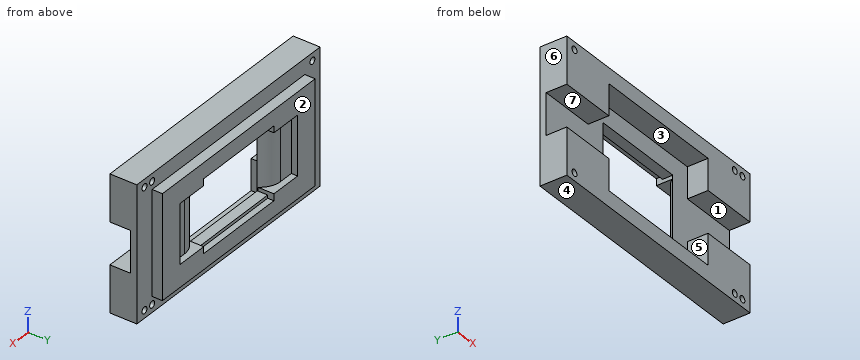
from build123d import *

# Parameters (mm, degrees)
BOSS_EXTRUDE3_DEPTH = 2
SKETCH1_6_W         = 100
SKETCH1_6_H         = 50
BOSS_EXTRUDE4_DEPTH = 5
SKETCH2_W           = 120
SKETCH2_H           = 65
SKETCH2_R           = 1.6
BOSS_EXTRUDE5_DEPTH = 13
SKETCH2_2_W         = 120
SKETCH2_2_H         = 65
SKETCH2_2_R         = 1.6
BOSS_EXTRUDE6_DEPTH = 3
CUT_EXTRUDE1_REACH  = 71.866
SKETCH7_W           = 43
SKETCH7_H           = 32
FILLET1_R           = 10
SKETCH8_W           = 38.5
SKETCH8_H           = 20
CUT_EXTRUDE2_DEPTH  = 10
SKETCH9_W           = 65
SKETCH9_H           = 50
CUT_EXTRUDE3_DEPTH  = 10


with BuildPart() as part:
    # Sketch1 → Boss-Extrude3 (new body)
    with BuildSketch(Plane(origin=(0, 0, 0), x_dir=(1, 0, 0), z_dir=(0, 1, 0))):
        Polygon((23, -14.25), (23, -17.5), (-23, -17.5), (-23, -14.25), (-38.5, -14.25), (-38.5, 14.25), (-23, 14.25), (-23, 17.5), (23, 17.5), (23, 14.25), (38.5, 14.25), (38.5, -14.25), align=None)
    extrude(amount=BOSS_EXTRUDE3_DEPTH)

    # Sketch1<6> → Boss-Extrude4 (add)
    with BuildSketch(Plane(origin=(0, 0, 0), x_dir=(1, 0, 0), z_dir=(0, 1, 0))):
        Rectangle(SKETCH1_6_W, SKETCH1_6_H)
        Polygon((23, -14.25), (23, -17.5), (-23, -17.5), (-23, -14.25), (-38.5, -14.25), (-38.5, 14.25), (-23, 14.25), (-23, 17.5), (23, 17.5), (23, 14.25), (38.5, 14.25), (38.5, -14.25), align=None, mode=Mode.SUBTRACT)
    extrude(amount=BOSS_EXTRUDE4_DEPTH)

    # Sketch2 → Boss-Extrude5 (add)
    with BuildSketch(Plane.XZ):
        Rectangle(SKETCH2_W, SKETCH2_H)
        with Locations(Location((-55, 28.75, 0), (0, 0, 90))):
            Circle(SKETCH2_R, mode=Mode.SUBTRACT)
        with Locations(Location((55, 28.75, 0), (0, 0, 90))):
            Circle(SKETCH2_R, mode=Mode.SUBTRACT)
        with Locations(Location((55, -28.75, 0), (0, 0, 90))):
            Circle(SKETCH2_R, mode=Mode.SUBTRACT)
        with Locations(Location((-55, -28.75, 0), (0, 0, 90))):
            Circle(SKETCH2_R, mode=Mode.SUBTRACT)
        with Locations(Location((50, 28.75, 0), (0, 0, 90))):
            Circle(SKETCH2_R, mode=Mode.SUBTRACT)
        with Locations(Location((50, -28.75, 0), (0, 0, 90))):
            Circle(SKETCH2_R, mode=Mode.SUBTRACT)
    extrude(amount=BOSS_EXTRUDE5_DEPTH)

    # Sketch2<2> → Boss-Extrude6 (add)
    with BuildSketch(Plane.XZ):
        Rectangle(SKETCH2_2_W, SKETCH2_2_H)
        with Locations(Location((-55, 28.75, 0), (0, 0, 90))):
            Circle(SKETCH2_2_R, mode=Mode.SUBTRACT)
        with Locations(Location((55, 28.75, 0), (0, 0, 90))):
            Circle(SKETCH2_2_R, mode=Mode.SUBTRACT)
        with Locations(Location((55, -28.75, 0), (0, 0, 90))):
            Circle(SKETCH2_2_R, mode=Mode.SUBTRACT)
        with Locations(Location((-55, -28.75, 0), (0, 0, 90))):
            Circle(SKETCH2_2_R, mode=Mode.SUBTRACT)
        with Locations(Location((50, 28.75, 0), (0, 0, 90))):
            Circle(SKETCH2_2_R, mode=Mode.SUBTRACT)
        with Locations(Location((50, -28.75, 0), (0, 0, 90))):
            Circle(SKETCH2_2_R, mode=Mode.SUBTRACT)
    extrude(amount=BOSS_EXTRUDE6_DEPTH)

    # Sketch7 → Cut-Extrude1 (cut, up to next)
    with BuildSketch(Plane(origin=(0, 2, 0), x_dir=(1, 0, 0), z_dir=(0, 1, 0)), mode=Mode.PRIVATE) as cut_extrude1_sk1:
        Rectangle(SKETCH7_W, SKETCH7_H)
    cut_extrude1_tool1 = extrude(cut_extrude1_sk1.sketch, amount=-CUT_EXTRUDE1_REACH, mode=Mode.PRIVATE) & part.part
    add(cut_extrude1_tool1.solids().sort_by_distance((0, 2, 0))[0], mode=Mode.SUBTRACT)

    # Fillet1
    # the kernel refuses this fillet: 10 mm, written as the material it takes off along each edge
    with BuildSketch(Plane(origin=(-21.5, 2, 16), x_dir=(0, -1, 0), z_dir=(0, 0, -1))) as fillet1_piece_1_section:
        with BuildLine():
            CenterArc((FILLET1_R, FILLET1_R), FILLET1_R, 180, 90)
            Line((0, FILLET1_R), (0, 0))
            Line((0, 0), (FILLET1_R, 0))
        make_face()
    fillet1_piece_1 = extrude(amount=32, mode=Mode.PRIVATE)
    fillet1_piece_1 = split(fillet1_piece_1, bisect_by=Plane(origin=(-23, -2.387167078, 15.125), z_dir=(1, 0, 0)), keep=Keep.TOP, mode=Mode.PRIVATE)
    add(fillet1_piece_1, mode=Mode.SUBTRACT)
    with BuildSketch(Plane(origin=(-21.5, 2, 41), x_dir=(0, -1, 0), z_dir=(0, 0, -1))) as fillet1_piece_2_section:
        with BuildLine():
            CenterArc((FILLET1_R, FILLET1_R), FILLET1_R, 180, 90)
            Line((0, FILLET1_R), (0, 0))
            Line((0, 0), (FILLET1_R, 0))
        make_face()
    fillet1_piece_2 = extrude(amount=82, mode=Mode.PRIVATE)
    fillet1_piece_2 = split(fillet1_piece_2, bisect_by=Plane(origin=(-23.780995079, -0.852225246, -14.25), z_dir=(0, 0, 1)), keep=Keep.TOP, mode=Mode.PRIVATE)
    fillet1_piece_2 = split(fillet1_piece_2, bisect_by=Plane(origin=(-23.780995079, -0.852225246, 14.25), z_dir=(0, 0, -1)), keep=Keep.TOP, mode=Mode.PRIVATE)
    add(fillet1_piece_2, mode=Mode.SUBTRACT)
    with BuildSketch(Plane(origin=(21.5, 2, -16), x_dir=(0, -1, 0), z_dir=(0, 0, 1))) as fillet1_piece_3_section:
        with BuildLine():
            CenterArc((FILLET1_R, FILLET1_R), FILLET1_R, 180, 90)
            Line((0, FILLET1_R), (0, 0))
            Line((0, 0), (FILLET1_R, 0))
        make_face()
    fillet1_piece_3 = extrude(amount=32, mode=Mode.PRIVATE)
    fillet1_piece_3 = split(fillet1_piece_3, bisect_by=Plane(origin=(23, -2.387167078, -15.125), z_dir=(-1, 0, 0)), keep=Keep.TOP, mode=Mode.PRIVATE)
    add(fillet1_piece_3, mode=Mode.SUBTRACT)
    with BuildSketch(Plane(origin=(21.5, 2, -41), x_dir=(0, -1, 0), z_dir=(0, 0, 1))) as fillet1_piece_4_section:
        with BuildLine():
            CenterArc((FILLET1_R, FILLET1_R), FILLET1_R, 180, 90)
            Line((0, FILLET1_R), (0, 0))
            Line((0, 0), (FILLET1_R, 0))
        make_face()
    fillet1_piece_4 = extrude(amount=82, mode=Mode.PRIVATE)
    fillet1_piece_4 = split(fillet1_piece_4, bisect_by=Plane(origin=(23.780995079, -0.852225246, 14.25), z_dir=(0, 0, -1)), keep=Keep.TOP, mode=Mode.PRIVATE)
    fillet1_piece_4 = split(fillet1_piece_4, bisect_by=Plane(origin=(23.780995079, -0.852225246, -14.25), z_dir=(0, 0, 1)), keep=Keep.TOP, mode=Mode.PRIVATE)
    add(fillet1_piece_4, mode=Mode.SUBTRACT)

    # Sketch8 → Cut-Extrude2 (cut)
    with BuildSketch(Plane.XZ.offset(13)):
        with Locations((-40.75, 0)):
            Rectangle(SKETCH8_W, SKETCH8_H)
        with Locations((40.75, 0)):
            Rectangle(SKETCH8_W, SKETCH8_H)
    extrude(amount=-CUT_EXTRUDE2_DEPTH, mode=Mode.SUBTRACT)

    # Sketch9 → Cut-Extrude3 (cut)
    with BuildSketch(Plane(origin=(0, -13, 0), x_dir=(-1, 0, 0), z_dir=(0, -1, 0))):
        Rectangle(SKETCH9_W, SKETCH9_H)
    extrude(amount=-CUT_EXTRUDE3_DEPTH, mode=Mode.SUBTRACT)


solid = part.part
Geometry: final body of the model. Coordinates: model frame, mm. Face numbers are marked on the shaded views. A direction names the side the tool comes from. Coordinates: 2 decimals unless noted, no trailing zeros. Write each loop counter-clockwise with the first axis right and the second up, starting at its lowest first coordinate (ties: lowest second). Pieces come first, ordered by that corner, then holes. Notation, with made-up numbers: (67.5, 26) - (72.5, 26) arc R35 cw to (72.5, 60) - close; hole circle Ø2 at (-19.5, 57.5). An arc over 180 degrees is marked (long way). Return JSON: item names as keys, results as strings.
Item 1: Pull-direction query (Z, two-part tool) for the marked faces 4, 5, 6 and 7; classes: +Z half, -Z half, draft (parallel to the pull), parting line (faces both ways), or undercut.
Completed:
{"face 4": "-Z half", "face 5": "undercut", "face 6": "draft", "face 7": "undercut"}
Item 2: Section query C-C (z = 28.75). Output: boundary loops of the cut face in (x, y).
Completed:
{"outline": "(-60, -13) - (-56.6, -13) - (-56.6, 0) - (-60, 0) - close; (-53.4, -13) - (48.4, -13) - (48.4, 0) - (-53.4, 0) - close; (51.6, -13) - (53.4, -13) - (53.4, 0) - (51.6, 0) - close; (56.6, -13) - (60, -13) - (60, 0) - (56.6, 0) - close"}
Item 3: Pin query (flat end, axial travel): pin 1 Ø3 at (x, z) = (-55, -28.75) entering from -Y; pin 2 Ø2.5 at (y, z) = (4, 1) entering from -X; pin 3 Ø1.2 at (x, z) = (2.5, 16.5) entering from +Y; pin 4 Ø2.5 at (x, y) = (6, 2.5) entering from -Z. Return the tip coordinate at first contact, or that it passes through.
Completed:
{"pin 1": "passes through", "pin 2": "stops at x = -50", "pin 3": "stops at y = 2", "pin 4": "stops at z = -25"}
Item 4: Section query B-B (x = -1.5). Output: boundary loops of the cut face in (y, z).
Completed:
{"outline": "(-13, -32.5) - (0, -32.5) - (0, -25) - (5, -25) - (5, -17.5) - (2, -17.5) - (2, -16) - (-3, -16) - (-3, -25) - (-13, -25) - close; (-13, 25) - (-3, 25) - (-3, 16) - (2, 16) - (2, 17.5) - (5, 17.5) - (5, 25) - (0, 25) - (0, 32.5) - (-13, 32.5) - close"}
Item 5: Reachability of the marked faces 1, 2 and 3 from +Z, -Z, +X, -X, +Y, -Y: full face, straight path, thin tool, end or side. Return the list, or none.
Completed:
{"face 1": "+X, -X, -Y", "face 2": "+Z, -Z, +X, -X, +Y", "face 3": "-Y"}
Item 6: Section query A-A (y = -6.5). Output: boundary loops of the cut face in (x, z), and give its area (3 significant figures).
Completed:
{"outline": "(-60, -32.5) - (60, -32.5) - (60, -10) - (32.5, -10) - (32.5, -25) - (-32.5, -25) - (-32.5, -10) - (-60, -10) - close; (-60, 10) - (-32.5, 10) - (-32.5, 25) - (32.5, 25) - (32.5, 10) - (60, 10) - (60, 32.5) - (-60, 32.5) - close; hole circle Ø3.2 at (-55, -28.75); hole circle Ø3.2 at (-55, 28.75); hole circle Ø3.2 at (50, -28.75); hole circle Ø3.2 at (50, 28.75); hole circle Ø3.2 at (55, -28.75); hole circle Ø3.2 at (55, 28.75)", "area": "3,400 mm2"}
Item 7: Line query: L1, parallel to X at y = -2.5, z = -28.75; L2, parallel to Z at x = 55, y = -6.5; L3, parallel to Z at x = -4, y = -2.5. Output: solid intervals per line, ascending.
Completed:
{"L1": "x = -60 to -56.6, -53.4 to 48.4, 51.6 to 53.4, 56.6 to 60", "L2": "z = -32.5 to -30.35, -27.15 to -10, 10 to 27.15, 30.35 to 32.5", "L3": "z = -32.5 to -16, 16 to 32.5"}
Item 8: Section query D-D (z = 7). Output: boundary loops of the cut face in (x, y).
Completed:
{"outline": "(-60, -3) - (-22.84, -3) arc R10 ccw to (-31.5, 2) - (-38.5, 2) - (-38.5, 5) - (-50, 5) - (-50, 0) - (-60, 0) - close; (22.84, -3) - (60, -3) - (60, 0) - (50, 0) - (50, 5) - (38.5, 5) - (38.5, 2) - (31.5, 2) arc R10 ccw to start"}
